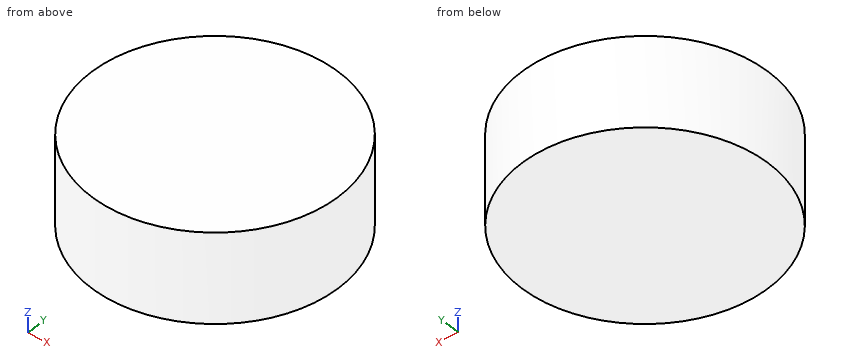
from build123d import *

# Parameters (mm, degrees)
F0_R      = 35
F1_DEPTH  = 25.4
F1_FACE_R = 35
F2_DEPTH  = 8
F3_DEPTH  = 10


with BuildPart() as f1:
    # F0 (on Top) → F1 (new body)
    with BuildSketch(Plane.XY):
        Circle(F0_R)
    extrude(amount=F1_DEPTH)

    # F1_face (on face) → F2 (join)
    with BuildSketch(Plane.XY.offset(25.4)):
        Circle(F1_FACE_R)
    extrude(amount=-F2_DEPTH)

    # F1_face (on face) → F3 (join)
    with BuildSketch(Plane.XY.offset(25.4)):
        Circle(F1_FACE_R)
    extrude(amount=-F3_DEPTH)


solid = f1.part
Design review of the part built by this model. Coordinates are the model's own, in mm. Give positions to 0.01 mm unless a question says otherwise; leave off trailing zeros. Loops run counter-clockwise (first coordinate to the right, second up) from the corner with the lowest first, then second, coordinate; pieces in that order, holes last. Notation, with made-up numbers: M 79,57 L 131,57 A26 ccw 131,76 Z; hole C 46.25,15 d3. An arc over 180 degrees is marked long. Write item = value, one per line.
Q1. We need section A-A (z = 12.5). Give the boundary of the cut face in (x, y), plus the area to 3 significant figures.
Output values:
outline = C 0,0 d70
area = 3,850 mm^2
Q2. We need section B-B (x = -25). Give the boundary of the cut face in (y, z).
Output values:
outline = M -24.49,0 L 24.49,0 L 24.49,25.4 L -24.49,25.4 Z
Q3. To check wall thickness, follow line 1 (X direction, y = 11, z = 16.25); line 2 (Y direction, x = 17, z = 10.5); line 3 (X direction, y = -17.5, z = 24). State the ranges of each line that lie inside material, in increasing order. Write a range as [from, to].
Output values:
line_1 = [-33.23, 33.23]
line_2 = [-30.59, 30.59]
line_3 = [-30.31, 30.31]
Q4. Insertion check: pin 1 (5 mm diameter, centred on x = -13, y = -8.5, fed in from -Z); pin 2 (2 mm diameter, centred on y = 17.5, z = 17, fed in from +X); pin 3 (1.5 mm diameter, centred on x = -18.5, z = 9.5, fed in from -Y); pin 4 (1 mm diameter, centred on y = -17, z = 22.5, fed in from -X). Each pin has a flat end and moves straight along its axis. Give the tip position at first contact, or say it passes through.
Output values:
pin_1 = 0
pin_2 = 30.87
pin_3 = -30.17
pin_4 = -30.87
Q5. We need section C-C (y = -29). Give the boundary of the cut face in (x, z), plus the area to 3 significant figures.
Output values:
outline = M -19.6,0 L 19.6,0 L 19.6,25.4 L -19.6,25.4 Z
area = 995 mm^2
